The listing builds one solid part. Answer for the finished solid, in the listing's coordinates (mm). Round coordinates to 2 decimals unless told otherwise and drop trailing zeros. Write each loop counter-clockwise with the first axis right and the second up, starting at its lowest first coordinate (ties: lowest second). Pieces come first, ordered by that corner, then holes.
from build123d import *

# Parameters (mm, degrees)
F0_W     = 40
F0_H     = 280
F0_R     = 12.5
F1_DEPTH = 5


with BuildPart() as f1:
    # F0 (on Front) → F1 (new body, symmetric)
    with BuildSketch(Plane.XZ):
        Rectangle(F0_W, F0_H)
        with Locations((0, -120)):
            Circle(F0_R, mode=Mode.SUBTRACT)
        Circle(F0_R, mode=Mode.SUBTRACT)
        with Locations((0, 120)):
            Circle(F0_R, mode=Mode.SUBTRACT)
    extrude(amount=F1_DEPTH, both=True)


solid = f1.part
1. Section A-A on z = -120 is taken. Determine the outline of the cut face in (x, y), plus the area to 3 significant figures.
Geometry says:
outline: (-20, -5) - (-12.5, -5) - (-12.5, 5) - (-20, 5) - close; (12.5, -5) - (20, -5) - (20, 5) - (12.5, 5) - close
area: 150 mm2
2. Section C-C on y = -1.5 is taken. Determine the outline of the cut face in (x, z), plus the area to 3 significant figures.
Geometry says:
outline: (-20, -140) - (20, -140) - (20, 140) - (-20, 140) - close; hole circle Ø25 at (0, -120); hole circle Ø25 at (0, 0); hole circle Ø25 at (0, 120)
area: 9,730 mm2
3. Section B-B on x = 0 is taken. Determine the outline of the cut face in (y, z), plus the area to 3 significant figures.
Geometry says:
outline: (-5, -140) - (5, -140) - (5, -132.5) - (-5, -132.5) - close; (-5, -107.5) - (5, -107.5) - (5, -12.5) - (-5, -12.5) - close; (-5, 12.5) - (5, 12.5) - (5, 107.5) - (-5, 107.5) - close; (-5, 132.5) - (5, 132.5) - (5, 140) - (-5, 140) - close
area: 2,050 mm2
4. Given pin 1 (20 mm diameter, centred on x = 0, z = 0, fed in from -Y), flat-ended and moving along its own axis, determine where the tip first touches the part or whether it passes through.
Geometry says:
pin 1: passes through
5. For a pull along X with two mould halves and no side action, classify faces 1 (the face through (0, 0, -140)), 2 (the face through (-20, 0, -2)), 3 (the face through (-1.627, 0.07, 132.394)) as released by +X, released by -X, zero draft, split by the parting line, or undercut.
Geometry says:
face 1: zero draft
face 2: released by -X
face 3: undercut
6. Straight lines are drawn through the part: line 1 along Z through (x, y) = (0, 3); line 2 along Z through (x, y) = (-7, -4); line 3 along X through (y, z) = (-4, -4). For each, find the intervals that lie inside material, in ascending order.
Geometry says:
line 1: z = -140 to -132.5, -107.5 to -12.5, 12.5 to 107.5, 132.5 to 140
line 2: z = -140 to -130.36, -109.64 to -10.36, 10.36 to 109.64, 130.36 to 140
line 3: x = -20 to -11.84, 11.84 to 20
